Read the model definition and answer for the solid it produces. Units are mm, in the model's axes. Face numbers are marked on the shaded views. Give positions to 0.01 mm unless a question says otherwise; leave off trailing zeros. Order: outer loops, then holes, each group sorted by start corner. A loop starts at its lowest first (then second) coordinate and runs counter-clockwise, first axis right, second up. Notation, with made-up numbers: (23.5, 42.25) - (54.5, 42.25) arc R13 cw to (54.5, 56.25) - close; hole circle Ø6 at (20.25, 32.5). An arc over 180 degrees is marked (long way). One line per item, written item: value. Start each with the question number.
```python
from build123d import *

# Parameters (mm, degrees)
BOSS_EXTRUDE1_DEPTH = 44.45
CUT_EXTRUDE2_DEPTH  = 254


with BuildPart() as part:
    # Sketch1 → Boss-Extrude1 (new body)
    with BuildSketch(Plane(origin=(0, 0, 0), x_dir=(1, 0, 0), z_dir=(0, 1, 0))):
        with BuildLine():
            Line((-253.572226701, 260.35), (0, 260.35))
            Line((0, 260.35), (0, 0))
            Line((0, 0), (-253.572226701, 0))
            ThreePointArc((-253.572226701, 0), (-285.75, 130.175), (-253.572226701, 260.35))
        make_face()
    extrude(amount=BOSS_EXTRUDE1_DEPTH)

    # Sketch2 → Cut-Extrude2 (cut)
    with BuildSketch(Plane.XY.offset(-3.175)):
        Polygon((-247.222226701, 41.275), (-215.252530753, 3.175), (32.837570188, 3.175), (32.837570188, 41.275), align=None)
    extrude(amount=-CUT_EXTRUDE2_DEPTH, mode=Mode.SUBTRACT)


solid = part.part
```
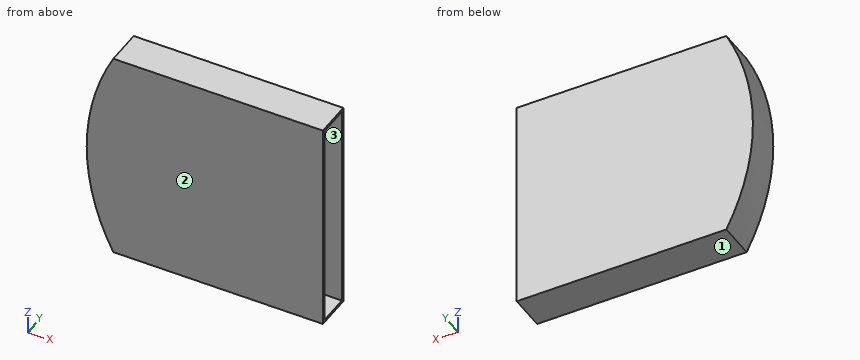
1) Section C-C on y = 20 is taken. Write down the section's boundary in (x, z) (3 decimals).
2) Each of these flat-tipped pins is pushed along its axis until it touches: pin 1 (2 mm diameter, centred on y = 24.5, z = -230.5, fed in from +X); pin 2 (8 mm diameter, centred on y = 25, z = -233.5, fed in from -X); pin 3 (1.5 mm diameter, centred on y = 17, z = -224, fed in from +X). Where does it stop, or does it pass through?
3) Find the intervals of material crossed by probe 1 along Z at (x, y) = (-222, 21.5) (3 decimals); probe 2 along Y at (x, z) = (-106.5, -37) (3 decimals); probe 3 along Y at (x, z) = (-239, -160) (3 decimals), in increasing order. Write a range as from..to.
4) Section B-B on z = -16.5 is taken. Write down the section's boundary in (x, y) (3 decimals).
5) Section A-A on x = -110 is taken. Write down the section's boundary in (y, z) (3 decimals), plus the area to 3 significant figures.
6) The mould has two halves that part along Z. Classify the marked faces 1, 2 and 3: +Z half, -Z half, draft (parallel to the pull), parting line (faces both ways), or undercut.
Solved:
1. outline: (-253.572, -260.35) - (0, -260.35) - (0, -257.175) - (-229.37, -257.175) - (-229.37, -3.175) - (0, -3.175) - (0, 0) - (-253.572, 0) arc R279.4 ccw to start
2. pin 1: stops at x = -232.31
2. pin 2: stops at x = -267.5
2. pin 3: stops at x = -226.22
3. probe 1: z = -260.35..-257.175, -3.175..0
3. probe 2: y = 0..3.175, 41.275..44.45
3. probe 3: y = 0..31.476, 41.275..44.45
4. outline: (-261.58, 0) - (0, 0) - (0, 3.175) - (-215.253, 3.175) - (-247.222, 41.275) - (0, 41.275) - (0, 44.45) - (-261.58, 44.45) - close
5. outline: (0, -260.35) - (44.45, -260.35) - (44.45, 0) - (0, 0) - close; hole (3.175, -257.175) - (41.275, -257.175) - (41.275, -3.175) - (3.175, -3.175) - close
5. area: 1,900 mm2
6. face 1: -Z half
6. face 2: draft
6. face 3: undercut
